from build123d import *

# Parameters (mm, degrees)
F0_W     = 49.15
F0_H     = 10.3
F0_R     = 1.65
F1_DEPTH = 5
F2_R     = 5


with BuildPart() as f1:
    # F0 (on Top) → F1 (new body)
    with BuildSketch(Plane.XY):
        Polygon((-29.575, 31.8), (-24.575, 31.8), (24.575, 31.8), (29.575, 31.8), (29.575, 46.7), (-29.575, 46.7), align=None)
        with BuildLine():
            ThreePointArc((-15.475, 38.45), (-17.125, 36.8), (-18.775, 38.45))
            Line((-18.775, 38.45), (-18.775, 40.05))
            ThreePointArc((-18.775, 40.05), (-17.125, 41.7), (-15.475, 40.05))
            Line((-15.475, 40.05), (-15.475, 38.45))
        make_face(mode=Mode.SUBTRACT)
        with BuildLine():
            ThreePointArc((18.775, 38.45), (17.125, 36.8), (15.475, 38.45))
            Line((15.475, 38.45), (15.475, 40.05))
            ThreePointArc((15.475, 40.05), (17.125, 41.7), (18.775, 40.05))
            Line((18.775, 40.05), (18.775, 38.45))
        make_face(mode=Mode.SUBTRACT)
        Polygon((29.575, 31.8), (24.575, 31.8), (24.575, 21.5), (24.575, -21.5), (24.575, -31.8), (29.575, -31.8), align=None)
        with Locations((0, 26.65)):
            Rectangle(F0_W, F0_H)
        with Locations((-17.125, 25.15)):
            Circle(F0_R, mode=Mode.SUBTRACT)
        with Locations((13.975, 25.15)):
            Circle(F0_R, mode=Mode.SUBTRACT)
        with Locations((0, -26.65)):
            Rectangle(F0_W, F0_H)
        with Locations((-17.125, -25.15)):
            Circle(F0_R, mode=Mode.SUBTRACT)
        with Locations((13.975, -25.15)):
            Circle(F0_R, mode=Mode.SUBTRACT)
        Polygon((-24.575, 21.5), (-24.575, 31.8), (-29.575, 31.8), (-29.575, -31.8), (-24.575, -31.8), (-24.575, -21.5), (-26.575, -21.5), (-26.575, 21.5), align=None)
        Polygon((-24.575, -31.8), (-29.575, -31.8), (-29.575, -46.7), (29.575, -46.7), (29.575, -31.8), (24.575, -31.8), align=None)
        with BuildLine():
            ThreePointArc((-18.775, -38.45), (-17.125, -36.8), (-15.475, -38.45))
            Line((-15.475, -38.45), (-15.475, -40.05))
            ThreePointArc((-15.475, -40.05), (-17.125, -41.7), (-18.775, -40.05))
            Line((-18.775, -40.05), (-18.775, -38.45))
        make_face(mode=Mode.SUBTRACT)
        with BuildLine():
            ThreePointArc((18.775, -40.05), (17.125, -41.7), (15.475, -40.05))
            Line((15.475, -40.05), (15.475, -38.45))
            ThreePointArc((15.475, -38.45), (17.125, -36.8), (18.775, -38.45))
            Line((18.775, -38.45), (18.775, -40.05))
        make_face(mode=Mode.SUBTRACT)
    extrude(amount=F1_DEPTH)

    # F2
    f2_edges = [f1.edges().sort_by_distance(p)[0] for p in [
        (29.575, 46.7, 2.5),
        (-29.575, 46.7, 2.5),
        (-29.575, -46.7, 2.5),
        (29.575, -46.7, 2.5),
    ]]
    fillet(f2_edges, radius=F2_R)


solid = f1.part
Geometry: final body of the model. Coordinates: model frame, mm. A direction names the side the tool comes from. Round coordinates to 2 decimals unless told otherwise and drop trailing zeros. Order: outer loops, then holes, each group sorted by start corner. A loop starts at its lowest first (then second) coordinate and runs counter-clockwise, first axis right, second up.
Q1. Material intervals for probe 1 along X at (y, z) = (-38.5, 1.5) (3 decimals); probe 2 along Y at (x, z) = (21, 3.6); probe 3 along X at (y, z) = (18, 2.8) (3 decimals), sorted ascending.
Result sheet:
probe 1: x = -29.575 to -18.775, -15.475 to 15.475, 18.775 to 29.575
probe 2: y = -46.7 to -21.5, 21.5 to 46.7
probe 3: x = -29.575 to -26.575, 24.575 to 29.575
Q2. Section C-C, the plane y = -8. Output: boundary loops of the cut face in (x, z) (3 decimals).
Result sheet:
outline: (-29.575, 0) - (-26.575, 0) - (-26.575, 5) - (-29.575, 5) - close; (24.575, 0) - (29.575, 0) - (29.575, 5) - (24.575, 5) - close
Q3. Section A-A, the plane x = -11.5. Output: boundary loops of the cut face in (y, z).
Result sheet:
outline: (-46.7, 0) - (-21.5, 0) - (-21.5, 5) - (-46.7, 5) - close; (21.5, 0) - (46.7, 0) - (46.7, 5) - (21.5, 5) - close
Q4. Section D-D, the plane z = 2.6. Give the number of separate pieces and of enclosed holes in the cut face, and give its area (3 significant figures).
Result sheet:
separate pieces: 1
enclosed holes: 9
area: 3,210 mm2
Q5. Pin query (flat end, axial travel): pin 1 (2.5 mm diameter, centred on x = -17.125, y = -25.15, fed in from +Z). Return the tip coordinate at first contact, or that it passes through.
Result sheet:
pin 1: passes through
Q6. Section B-B, the plane y = -25.15. Output: boundary loops of the cut face in (x, z) (3 decimals).
Result sheet:
outline: (-29.575, 0) - (-18.775, 0) - (-18.775, 5) - (-29.575, 5) - close; (-15.475, 0) - (12.325, 0) - (12.325, 5) - (-15.475, 5) - close; (15.625, 0) - (29.575, 0) - (29.575, 5) - (15.625, 5) - close
Q7. Access query for faces 1 (the face through (26, 1, 5)), 2 (the face through (-17.1, -41.7, 2.5)). Directions: +Z, -Z, +X, -X, +Y, -Y. A direction counts if a zero-diameter tool reaches every point of the face in a straight line with its end or side. Return the directions, or none.
Result sheet:
face 1: +Z, +X, -X, +Y, -Y
face 2: +Z, -Z
Q8. Mould query, pull axis X, two halves, no side actions, for faces 3 (the face through (26, 1, 0)), 4 (the face through (29.575, -1, 2)), 5 (the face through (17.2, 36.8, 2.5)). Classes: released by +X, released by -X, zero draft, split by the parting line, or undercut.
Result sheet:
face 3: zero draft
face 4: released by +X
face 5: undercut
